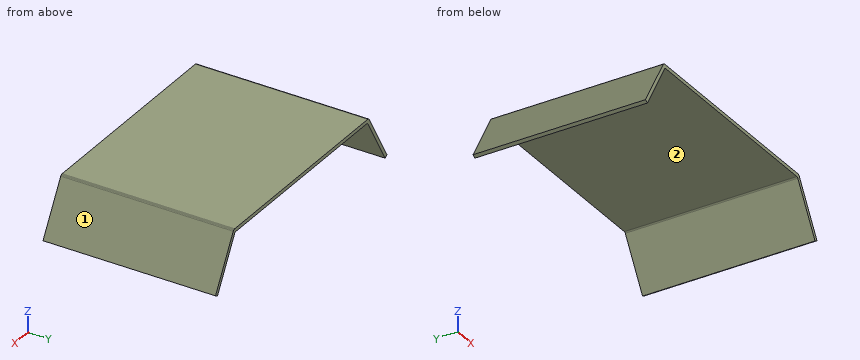
```python
from build123d import *

# Parameters (mm, degrees)
BOSS_EXTRUDE1_DEPTH = 152.4
FILLET1_R           = 1.5875


with BuildPart() as part:
    # Sketch1 → Boss-Extrude1 (new body)
    with BuildSketch(Plane(origin=(0, 0, 0), x_dir=(1, 0, 0), z_dir=(0, 1, 0))):
        Polygon((94.7975625, -1.5875), (-94.7975625, -1.5875), (-96.172377829, -0.79375), (-121.572377829, 43.200340512), (-118.822747171, 44.787840512), (-93.881018948, 1.5875), (93.881018948, 1.5875), (118.822747171, 44.787840512), (121.572377829, 43.200340512), (96.172377829, -0.79375), align=None)
    extrude(amount=BOSS_EXTRUDE1_DEPTH)

    # Fillet1
    fillet1_edges = [part.edges().sort_by_distance(p)[0] for p in [
        (94.7975625, 76.2, 1.5875),
        (-94.7975625, 76.2, 1.5875),
        (-96.172377829, 76.2, 0.79375),
        (-93.881018948, 76.2, -1.5875),
        (93.881018948, 76.2, -1.5875),
        (96.172377829, 76.2, 0.79375),
    ]]
    fillet(fillet1_edges, radius=FILLET1_R)


solid = part.part
```
For this review, take the finished solid that the model builds, in its own axes (mm). Face numbers are marked on the shaded views. A direction names the side the tool comes from. Coordinates: 2 decimals unless noted, no trailing zeros. Write each loop counter-clockwise with the first axis right and the second up, starting at its lowest first coordinate (ties: lowest second). Pieces come first, ordered by that corner, then holes.
(1) Add section B-B on z = -7.5. Give the boundary of the cut face in (x, y), then the cut area to 3 significant figures.
(2) For pin 1 Ø6 at (y, z) = (108.5, -16.5) entering from +X; pin 2 Ø6 at (x, y) = (75, 28.5) entering from -Z; pin 3 Ø2 at (y, z) = (129, -19.5) entering from -X, all flat-tipped, find the tip position at first contact; note any pin that passes through.
(3) Tool access review of the marked faces 1 and 2: name each direction out of +Z, -Z, +X, -X, +Y, -Y from which nothing blocks a thin tool from reaching the whole face with its end or side.
(4) Add section C-C on x = 31. Give the boundary of the cut face in (y, z).
(5) Add section A-A on y = 143. Give the boundary of the cut face in (x, z) (1 decimal), then the cut area to 3 significant figures.
(6) Wall thickness on probe 1 along X at (y, z) = (8.5, -21) (3 decimals); probe 2 along X at (y, z) = (14.5, -10.5); probe 3 along Z at (x, y) = (21.5, 7.5): over which ranges is each line inside the solid? List them lowest first.
Answer sheet:
1. outline: (-100.96, 0) - (-97.29, 0) - (-97.29, 152.4) - (-100.96, 152.4) - close; (97.29, 0) - (100.96, 0) - (100.96, 152.4) - (97.29, 152.4) - close
1. area: 1,120 mm2
2. pin 1: stops at x = 107.89
2. pin 2: stops at z = -1.59
2. pin 3: stops at x = -108.47
3. face 1: +Z, +X, +Y, -Y
3. face 2: -Z, +Y, -Y
4. outline: (0, -1.59) - (152.4, -1.59) - (152.4, 1.59) - (0, 1.59) - close
5. outline: (-121.6, -43.2) - (-118.8, -44.8) - (-94.3, -2.4) arc R1.6 cw to (-93, -1.6) - (93, -1.6) arc R1.6 cw to (94.3, -2.4) - (118.8, -44.8) - (121.6, -43.2) - (96.4, 0.4) arc R1.6 ccw to (95.8, 1) - (95.2, 1.4) arc R1.6 ccw to (94.4, 1.6) - (-94.4, 1.6) arc R1.6 ccw to (-95.2, 1.4) - (-95.8, 1) arc R1.6 ccw to (-96.4, 0.4) - close
5. area: 924 mm2
6. probe 1: x = -108.755 to -105.089, 105.089 to 108.755
6. probe 2: x = -102.69 to -99.03, 99.03 to 102.69
6. probe 3: z = -1.59 to 1.59
